from build123d import *

# Parameters (mm, degrees)
F0_W     = 45
F0_H     = 79
F0_R     = 3.75
F0_R_2   = 4
F0_R_3   = 1.75
F0_R_4   = 2.25
F1_DEPTH = 4
F2_DEPTH = 2
F3_R     = 5
F4_DEPTH = 2


with BuildPart() as f1:
    # F0 (on Front) → F1 (new body)
    with BuildSketch(Plane.XZ):
        Rectangle(F0_W, F0_H)
        with Locations((-9, -34.5)):
            Circle(F0_R, mode=Mode.SUBTRACT)
        with Locations((-17.5, -17.5)):
            Circle(F0_R_2, mode=Mode.SUBTRACT)
        with Locations((-9, -10.5)):
            Circle(F0_R, mode=Mode.SUBTRACT)
        with Locations((9, -34.5)):
            Circle(F0_R, mode=Mode.SUBTRACT)
        with Locations((9, -10.5)):
            Circle(F0_R, mode=Mode.SUBTRACT)
        with Locations((17.5, -17.5)):
            Circle(F0_R_2, mode=Mode.SUBTRACT)
        with Locations((-17.5, 0)):
            Circle(F0_R_3, mode=Mode.SUBTRACT)
        with Locations((-17.5, 17.5)):
            Circle(F0_R_2, mode=Mode.SUBTRACT)
        with BuildLine():
            ThreePointArc((-5.25, 10.5), (-12.354102, 8.822949), (-6.75, 13.5))
            ThreePointArc((-6.75, 13.5), (-5.645898, 12.177051), (-5.25, 10.5))
        make_face(mode=Mode.SUBTRACT)
        with BuildLine():
            ThreePointArc((-5.25, 34.5), (-5.645898, 32.822949), (-6.75, 31.5))
            ThreePointArc((-6.75, 31.5), (-12.354102, 36.177051), (-5.25, 34.5))
        make_face(mode=Mode.SUBTRACT)
        Circle(F0_R_2, mode=Mode.SUBTRACT)
        with BuildLine():
            ThreePointArc((12.75, 10.5), (7.322949, 7.145898), (6.75, 13.5))
            ThreePointArc((6.75, 13.5), (10.677051, 13.854102), (12.75, 10.5))
        make_face(mode=Mode.SUBTRACT)
        with Locations((17.5, 0)):
            Circle(F0_R_3, mode=Mode.SUBTRACT)
        with Locations((17.5, 17.5)):
            Circle(F0_R_2, mode=Mode.SUBTRACT)
        with BuildLine():
            ThreePointArc((12.75, 34.5), (10.677051, 31.145898), (6.75, 31.5))
            ThreePointArc((6.75, 31.5), (7.322949, 37.854102), (12.75, 34.5))
        make_face(mode=Mode.SUBTRACT)
        with BuildLine():
            ThreePointArc((-7.65, 32.7), (-6.987539, 33.493769), (-6.75, 34.5))
            ThreePointArc((-6.75, 34.5), (-11.012461, 35.506231), (-7.65, 32.7))
        make_face()
        with BuildLine():
            ThreePointArc((-5.25, 34.5), (-12.354102, 36.177051), (-6.75, 31.5))
            ThreePointArc((-6.75, 31.5), (-5.645898, 32.822949), (-5.25, 34.5))
        make_face()
        with BuildLine():
            ThreePointArc((-7.65, 32.7), (-11.012461, 35.506231), (-6.75, 34.5))
            ThreePointArc((-6.75, 34.5), (-6.987539, 33.493769), (-7.65, 32.7))
        make_face(mode=Mode.SUBTRACT)
        with BuildLine():
            ThreePointArc((11.25, 34.5), (7.993769, 36.512461), (7.65, 32.7))
            ThreePointArc((7.65, 32.7), (10.006231, 32.487539), (11.25, 34.5))
        make_face()
        with BuildLine():
            ThreePointArc((12.75, 34.5), (7.322949, 37.854102), (6.75, 31.5))
            ThreePointArc((6.75, 31.5), (10.677051, 31.145898), (12.75, 34.5))
        make_face()
        with BuildLine():
            ThreePointArc((11.25, 34.5), (10.006231, 32.487539), (7.65, 32.7))
            ThreePointArc((7.65, 32.7), (7.993769, 36.512461), (11.25, 34.5))
        make_face(mode=Mode.SUBTRACT)
        with BuildLine():
            ThreePointArc((11.25, 10.5), (10.006231, 12.512461), (7.65, 12.3))
            ThreePointArc((7.65, 12.3), (7.993769, 8.487539), (11.25, 10.5))
        make_face()
        with BuildLine():
            ThreePointArc((12.75, 10.5), (10.677051, 13.854102), (6.75, 13.5))
            ThreePointArc((6.75, 13.5), (7.322949, 7.145898), (12.75, 10.5))
        make_face()
        with BuildLine():
            ThreePointArc((11.25, 10.5), (7.993769, 8.487539), (7.65, 12.3))
            ThreePointArc((7.65, 12.3), (10.006231, 12.512461), (11.25, 10.5))
        make_face(mode=Mode.SUBTRACT)
        with BuildLine():
            ThreePointArc((-6.75, 10.5), (-6.987539, 11.506231), (-7.65, 12.3))
            ThreePointArc((-7.65, 12.3), (-11.012461, 9.493769), (-6.75, 10.5))
        make_face()
        with BuildLine():
            ThreePointArc((-5.25, 10.5), (-5.645898, 12.177051), (-6.75, 13.5))
            ThreePointArc((-6.75, 13.5), (-12.354102, 8.822949), (-5.25, 10.5))
        make_face()
        with BuildLine():
            ThreePointArc((-6.75, 10.5), (-11.012461, 9.493769), (-7.65, 12.3))
            ThreePointArc((-7.65, 12.3), (-6.987539, 11.506231), (-6.75, 10.5))
        make_face(mode=Mode.SUBTRACT)
        with Locations((-17.5, 17.5)):
            Circle(F0_R_2)
        with Locations((-17.5, 17.5)):
            Circle(F0_R_3, mode=Mode.SUBTRACT)
        Circle(F0_R_2)
        with Locations((-17.5, -17.5)):
            Circle(F0_R_2)
        with Locations((-17.5, -17.5)):
            Circle(F0_R_3, mode=Mode.SUBTRACT)
        with Locations((17.5, -17.5)):
            Circle(F0_R_2)
        with Locations((17.5, -17.5)):
            Circle(F0_R_3, mode=Mode.SUBTRACT)
        with Locations((17.5, 17.5)):
            Circle(F0_R_2)
        with Locations((17.5, 17.5)):
            Circle(F0_R_3, mode=Mode.SUBTRACT)
        with Locations((9, -10.5)):
            Circle(F0_R)
        with Locations((9, -10.5)):
            Circle(F0_R_4, mode=Mode.SUBTRACT)
        with Locations((-9, -10.5)):
            Circle(F0_R)
        with Locations((-9, -10.5)):
            Circle(F0_R_4, mode=Mode.SUBTRACT)
        with Locations((9, -34.5)):
            Circle(F0_R)
        with Locations((9, -34.5)):
            Circle(F0_R_4, mode=Mode.SUBTRACT)
        with Locations((-9, -34.5)):
            Circle(F0_R)
        with Locations((-9, -34.5)):
            Circle(F0_R_4, mode=Mode.SUBTRACT)
    extrude(amount=F1_DEPTH)

    # F0 (on Front) → F2 (join)
    with BuildSketch(Plane.XZ):
        with Locations((-17.5, 17.5)):
            Circle(F0_R_2)
        with Locations((-17.5, 17.5)):
            Circle(F0_R_3, mode=Mode.SUBTRACT)
        with Locations((17.5, 17.5)):
            Circle(F0_R_2)
        with Locations((17.5, 17.5)):
            Circle(F0_R_3, mode=Mode.SUBTRACT)
        Circle(F0_R_2)
        with Locations((-17.5, -17.5)):
            Circle(F0_R_2)
        with Locations((-17.5, -17.5)):
            Circle(F0_R_3, mode=Mode.SUBTRACT)
        with Locations((17.5, -17.5)):
            Circle(F0_R_2)
        with Locations((17.5, -17.5)):
            Circle(F0_R_3, mode=Mode.SUBTRACT)
    extrude(amount=-F2_DEPTH)

    # F3
    f3_edges = [f1.edges().sort_by_distance(p)[0] for p in [
        (-22.5, -2, 39.5),
        (-22.5, -2, -39.5),
        (22.5, -2, -39.5),
        (22.5, -2, 39.5),
    ]]
    fillet(f3_edges, radius=F3_R)

    # F0 (on Front) → F4 (cut)
    with BuildSketch(Plane.XZ):
        with BuildLine():
            ThreePointArc((-5.25, 34.5), (-12.354102, 36.177051), (-6.75, 31.5))
            ThreePointArc((-6.75, 31.5), (-5.645898, 32.822949), (-5.25, 34.5))
        make_face()
        with BuildLine():
            ThreePointArc((-7.65, 32.7), (-11.012461, 35.506231), (-6.75, 34.5))
            ThreePointArc((-6.75, 34.5), (-6.987539, 33.493769), (-7.65, 32.7))
        make_face(mode=Mode.SUBTRACT)
        with BuildLine():
            ThreePointArc((-5.25, 10.5), (-5.645898, 12.177051), (-6.75, 13.5))
            ThreePointArc((-6.75, 13.5), (-12.354102, 8.822949), (-5.25, 10.5))
        make_face()
        with BuildLine():
            ThreePointArc((-6.75, 10.5), (-11.012461, 9.493769), (-7.65, 12.3))
            ThreePointArc((-7.65, 12.3), (-6.987539, 11.506231), (-6.75, 10.5))
        make_face(mode=Mode.SUBTRACT)
        with BuildLine():
            ThreePointArc((12.75, 10.5), (10.677051, 13.854102), (6.75, 13.5))
            ThreePointArc((6.75, 13.5), (7.322949, 7.145898), (12.75, 10.5))
        make_face()
        with BuildLine():
            ThreePointArc((11.25, 10.5), (7.993769, 8.487539), (7.65, 12.3))
            ThreePointArc((7.65, 12.3), (10.006231, 12.512461), (11.25, 10.5))
        make_face(mode=Mode.SUBTRACT)
        with BuildLine():
            ThreePointArc((12.75, 34.5), (7.322949, 37.854102), (6.75, 31.5))
            ThreePointArc((6.75, 31.5), (10.677051, 31.145898), (12.75, 34.5))
        make_face()
        with BuildLine():
            ThreePointArc((11.25, 34.5), (10.006231, 32.487539), (7.65, 32.7))
            ThreePointArc((7.65, 32.7), (7.993769, 36.512461), (11.25, 34.5))
        make_face(mode=Mode.SUBTRACT)
        with Locations((-9, -10.5)):
            Circle(F0_R)
        with Locations((-9, -10.5)):
            Circle(F0_R_4, mode=Mode.SUBTRACT)
        with Locations((9, -10.5)):
            Circle(F0_R)
        with Locations((9, -10.5)):
            Circle(F0_R_4, mode=Mode.SUBTRACT)
        with Locations((9, -34.5)):
            Circle(F0_R)
        with Locations((9, -34.5)):
            Circle(F0_R_4, mode=Mode.SUBTRACT)
        with Locations((-9, -34.5)):
            Circle(F0_R)
        with Locations((-9, -34.5)):
            Circle(F0_R_4, mode=Mode.SUBTRACT)
    extrude(amount=F4_DEPTH, mode=Mode.SUBTRACT)


solid = f1.part
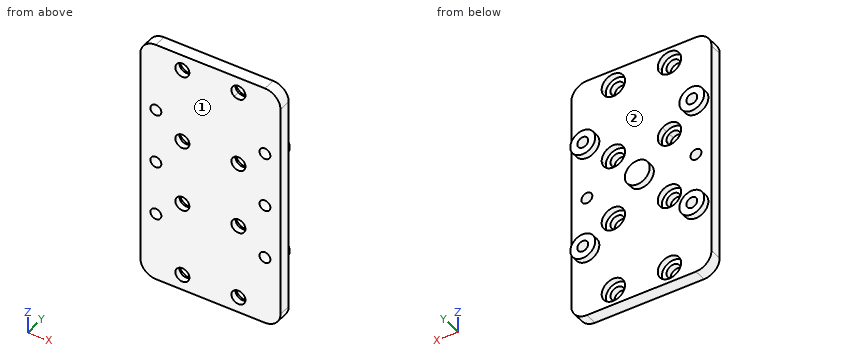
Geometry check sheet. Reference: the model listing, model coordinates, mm. Face numbers are marked on the shaded views. Round coordinates to 2 decimals unless told otherwise and drop trailing zeros. Loops run counter-clockwise (first coordinate to the right, second up) from the corner with the lowest first, then second, coordinate; pieces in that order, holes last.
Item 1: Gauge pin test, flat ends, axial feed: pin 1 (5 mm diameter, centred on x = 9, z = -10.5, fed in from +Y); pin 2 (8 mm diameter, centred on x = -8, z = -33, fed in from +Y). Record the tip position at first contact, or that the pin passes through.
Item 2: Mould release check, pull along X, two halves, no side actions. Record for the marked faces 1 and 2: pulls with the +X half, pulls with the -X half, needs draft (parallel to the pull), parting line crosses it, or undercut.
Item 3: Cross-section at B-B on y = -1.2. Count the separate pieces of the cut face and the enclosed holes in it, then the cut area to 3 significant figures.
Item 4: Cross-section at A-A on z = 17.5. Record the boundary of the cut face in (x, y).
Item 5: Cross-section at D-D on x = -1. Record the boundary of the cut face in (y, z).
Item 6: Thickness scan on line 1 (Z direction, x = -9, y = -3.1); line 2 (Z direction, x = 9, y = -0.9); line 3 (Z direction, x = -17.5, y = -1.1). Record the ranges inside material, lowest first.
Answer sheet:
1. pin 1: stops at y = -2
1. pin 2: stops at y = 0
2. face 1: needs draft
2. face 2: undercut
3. separate pieces: 1
3. enclosed holes: 14
3. area: 3,120 mm2
4. outline: (-22.5, -4) - (-19.25, -4) - (-19.25, 2) - (-21.5, 2) - (-21.5, 0) - (-22.5, 0) - close; (-15.75, -4) - (15.75, -4) - (15.75, 2) - (13.5, 2) - (13.5, 0) - (-13.5, 0) - (-13.5, 2) - (-15.75, 2) - close; (19.25, -4) - (22.5, -4) - (22.5, 0) - (21.5, 0) - (21.5, 2) - (19.25, 2) - close
5. outline: (-4, -39.5) - (0, -39.5) - (0, -3.87) - (2, -3.87) - (2, 3.87) - (0, 3.87) - (0, 39.5) - (-4, 39.5) - close
6. line 1: z = -39.5 to -36.75, -32.25 to -12.75, -8.25 to 8.25, 12.75 to 32.25, 36.75 to 39.5
6. line 2: z = -39.5 to -38.25, -30.75 to -14.25, -6.75 to 6.75, 14.25 to 30.75, 38.25 to 39.5
6. line 3: z = -39.5 to -19.25, -15.75 to -1.75, 1.75 to 15.75, 19.25 to 39.5
